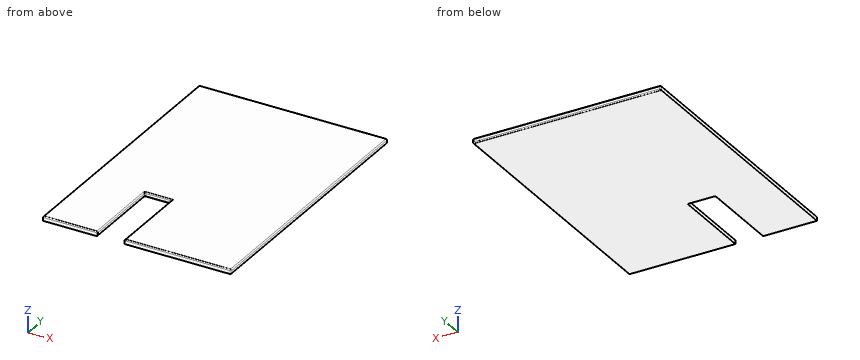
from build123d import *

# Parameters (mm, degrees)
BOSS_EXTRUDE1_DEPTH = 20
FILLET1_R           = 5


with BuildPart() as part:
    # Sketch1 → Boss-Extrude1 (new body)
    with BuildSketch(Plane.XY):
        Polygon((-175.5, -595), (-175.5, -235), (-55.5, -235), (-55.5, -595), (417.5, -595), (417.5, 595), (-417.5, 595), (-417.5, -595), align=None)
    extrude(amount=BOSS_EXTRUDE1_DEPTH)

    # Fillet1
    fillet1_edges = [part.edges().sort_by_distance(p)[0] for p in [
        (0, 595, 0),
        (417.5, 0, 0),
        (0, 595, 20),
        (-175.5, -235, 10),
        (-175.5, -595, 10),
        (-417.5, 595, 10),
        (417.5, 595, 10),
        (417.5, -595, 10),
        (-417.5, 0, 20),
        (-296.5, -595, 20),
        (-175.5, -415, 20),
        (-115.5, -235, 20),
        (-55.5, -415, 20),
        (181, -595, 20),
        (417.5, 0, 20),
        (-115.5, -235, 0),
        (-175.5, -415, 0),
    ]]
    fillet(fillet1_edges, radius=FILLET1_R)


solid = part.part
Verification items for the finished model (mm, model axes). Give positions to 0.01 mm unless a question says otherwise; leave off trailing zeros. Write each loop counter-clockwise with the first axis right and the second up, starting at its lowest first coordinate (ties: lowest second). Pieces come first, ordered by that corner, then holes. Notation, with made-up numbers: (78, 41.25) -> (88, 41.25) arc R36 ccw to (88, 76.25) -> close; hole circle Ø7 at (31, 70.5). An arc over 180 degrees is marked (long way). Use CSV: the item, a comma, the result in double quotes.
(1) Sectioned sample at A-A (z = 11.5). Record the cut outline in (x, y), plus the area to 3 significant figures.
Derived:
outline,"(-417.5, -595) -> (-180.5, -595) arc R5 ccw to (-175.5, -590) -> (-175.5, -240) arc R5 cw to (-170.5, -235) -> (-55.5, -235) -> (-55.5, -595) -> (412.5, -595) arc R5 ccw to (417.5, -590) -> (417.5, 590) arc R5 ccw to (412.5, 595) -> (-412.5, 595) arc R5 ccw to (-417.5, 590) -> close"
area,"950,000 mm^2"
(2) Go/stop test with a flat-tipped pin: pin 1 (11 mm diameter, centred on x = -131.5, z = 12, fed in from -Y). Record where the tip stops, or that it passes through.
Derived:
pin 1,"stops at y = -235"
(3) Sectioned sample at B-B (x = -140). Record the cut outline in (y, z), plus the area to 3 significant figures.
Derived:
outline,"(-235, 5) arc R5 ccw to (-230, 0) -> (590, 0) arc R5 ccw to (595, 5) -> (595, 15) arc R5 ccw to (590, 20) -> (-230, 20) arc R5 ccw to (-235, 15) -> close"
area,"16,600 mm^2"
(4) Material ranges on L1, parallel to X at y = -527, z = 8.5; L2, parallel to X at y = 1.5, z = 4.75; L3, parallel to Y at x = -167.5, z = 11, recorded low to high.
Derived:
L1,"x = -417.5 to -175.5, -55.5 to 417.5"
L2,"x = -417.5 to 417.49"
L3,"y = -235 to 595"
